Could you check a few things on this model? Use its own coordinates, in mm. Give positions to 0.01 mm unless a question says otherwise; leave off trailing zeros. Loops run counter-clockwise (first coordinate to the right, second up) from the corner with the lowest first, then second, coordinate; pieces in that order, holes last. Notation, with made-up numbers: (-5.5, 31.5) -> (14.5, 31.5) arc R22 cw to (14.5, 62.5) -> close; hole circle Ø10 at (56.25, -10). An arc over 180 degrees is marked (long way). Write each question's results on one line, items separated by ' | '. Start each with the question number.
Q1. If we section it at C-C, the plane y = 132.5: List the corners of the cut face in (x, z) for me.
Q2. If we section it at D-D, the plane x = 272.5: List the corners of the cut face in (y, z) for me.
Q3. If we section it at A-A, the plane x = -90: List the corners of the cut face in (y, z) for me.
Q4. If I drill on line 1 along X through (y, z) = (-28, 1.1); line 2 along X through (y, z) = (106, 0.75); line 3 along X through (y, z) = (-38, 1.25), over which ranges is the centre line in solid material (lowest first)?
Q5. If we section it at B-B, the plane z = 0.7: Give the number of separate pieces and of enclosed holes in the cut face, plus the area to 3 significant figures.
Q6. Will this pin go through, and if not, where does the flat tip stop? P1, Ø1.5, axis at y = -41, z = 2, coming from the -X side.
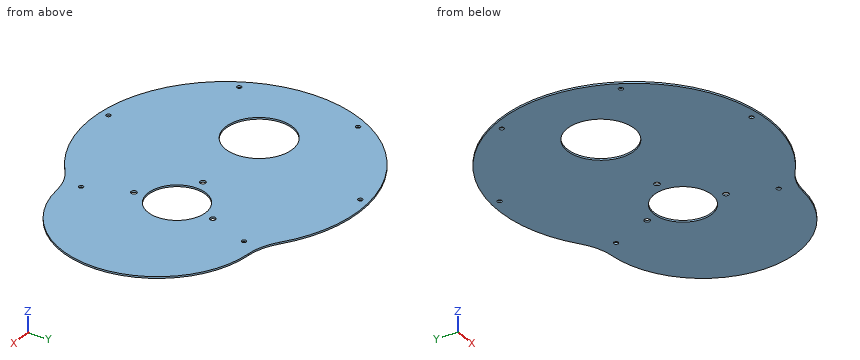
from build123d import *

# Parameters (mm, degrees)
F0_R            = 59
F0_R_2          = 51
F1_DEPTH        = 3
F2_R            = 100
F3_D            = 8
F3_COPIES_COUNT = 6
F3_COPIES_ANGLE = 280
F4_D            = 10


# Not quite as in the source:
# - a pattern or mirror of a feature is missing from the dataset's text; its kind, count and spacing are read off the source's solid


with BuildPart() as f1:
    # F0 (on Top) → F1 (new body)
    with BuildSketch(Plane.XY):
        with BuildLine():
            ThreePointArc((167.9378605318, -167.9378605318), (297.3413197874, -124.7660894685), (352.5, 0))
            ThreePointArc((352.5, 0), (297.3413197874, 124.7660894685), (167.9378605318, 167.9378605318))
            ThreePointArc((167.9378605318, 167.9378605318), (-237.5, 0), (167.9378605318, -167.9378605318))
        make_face()
        with Locations((-90, 0)):
            Circle(F0_R, mode=Mode.SUBTRACT)
        with Locations((131.5, 0)):
            Circle(F0_R_2, mode=Mode.SUBTRACT)
    extrude(amount=F1_DEPTH)

    # F2
    f2_edges = [f1.edges().sort_by_distance(p)[0] for p in [
        (167.937861, -167.937861, 1.5),
        (167.937861, 167.937861, 1.5),
    ]]
    fillet(f2_edges, radius=F2_R)

    # F3 (through all)
    with Locations(Plane(origin=(0, 0, 0), x_dir=(1, 0, 0), z_dir=(0, 0, -1))):
        with Locations((170.444888594, -143.0202431553)):
            f3 = Hole(F3_D / 2)

    # F3_copies: F3 ×6 about axis
    f3_copies_axis = Axis((0, 0, 0), (0, 0, 1))
    for i in range(1, F3_COPIES_COUNT):
        add(f3.rotate(f3_copies_axis, i * F3_COPIES_ANGLE / (F3_COPIES_COUNT - 1)), mode=Mode.SUBTRACT)

    # F4 (through all)
    with Locations(Plane(origin=(0, 0, 0), x_dir=(1, 0, 0), z_dir=(0, 0, -1))):
        with Locations((141.2421170672, -69.3187648119), (61.5, 0), (141.2421170672, 69.3187648119)):
            Hole(F4_D / 2)


solid = f1.part
Final values:
1) outline: (-197.1, 0) -> (288.21, 0) -> (288.21, 3) -> (-197.1, 3) -> close
2) outline: (-143.49, 0) -> (143.49, 0) -> (143.49, 3) -> (-143.49, 3) -> close
3) outline: (-219.79, 0) -> (-59, 0) -> (-59, 3) -> (-219.79, 3) -> close; (59, 0) -> (219.79, 0) -> (219.79, 3) -> (59, 3) -> close
4) line 1: x = -235.84 to -141.93, -38.07 to 88.87, 174.13 to 350.16 | line 2: x = -212.53 to -200.15, -192.77 to 315.04 | line 3: x = -234.44 to -135.13, -44.87 to 97.49, 165.51 to 348.16
5) separate pieces: 1 | enclosed holes: 11 | area: 192,000 mm²
6) P1: stops at x = -234.06
